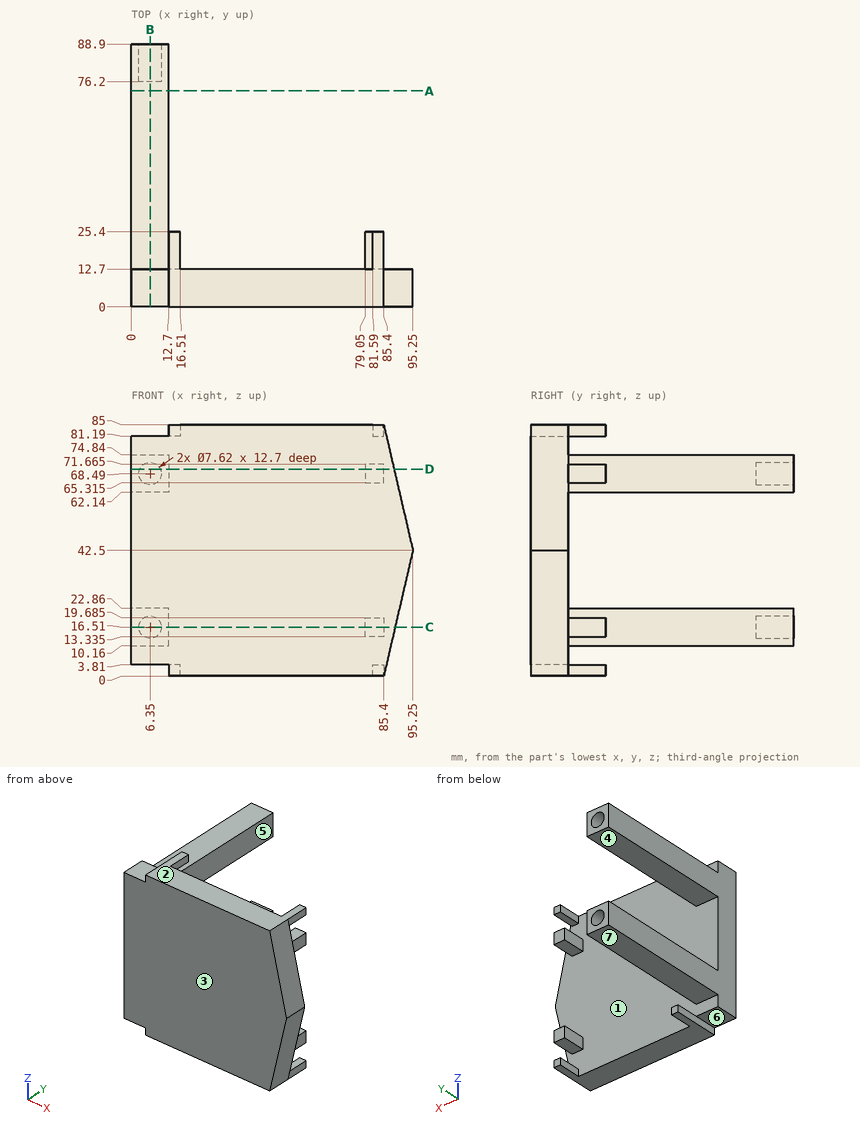
Answer from the drawing. Dimensions are ordinates in mm from the lowest x, y and z of the part. A direction names the side the tool comes from. Give positions to 0.01 mm unless a question says otherwise; leave off trailing zeros. Write each loop counter-clockwise with the first axis right and the second up, starting at its lowest first coordinate (ties: lowest second). Pieces come first, ordered by that corner, then holes.
1) A tool of negligible diameter and unlimited length cuts with its end or side. For the marked faces 5, 6 and 7, from which of +Z, -Z, +X, -X, +Y, -Y can it reach the whole face along a straight path? Write none if from no direction.
2) Section B-B (x = 6.35) is taken. Write down the section's boundary in (y, z), and give its area (3 significant figures).
3) Section D-D (z = 70) is taken. Write down the section's boundary in (x, y).
4) Section A-A (y = 73) is taken. Write down the section's boundary in (x, z).
5) For a pull along Z with two mould halves and no side action, classify the marked faces 1, 2, 3 and 4 as pulls with the +Z half, pulls with the -Z half, needs draft (parallel to the pull), parting line crosses it, or undercut.
6) Find the intervals of material crossed by L1, parallel to Z at x = 6, y = 83; L2, parallel to X at y = 83, z = 68; L3, parallel to Y at x = 37, z = 55.5, in increasing order.
7) Section C-C (z = 16.51) is taken. Write down the section's boundary in (x, y), and give its area (3 significant figures).
8) Given P1, Ø6, axis at x = 7.5, z = 16, coming from the +Y side; P2, Ø10, axis at x = 8, y = 39.5, coming from the -Z side; P3, Ø3, axis at x = 57, z = 21, coming from the +Y side; P4, Ø1.9, axis at y = 21.5, z = 83, coming from the -X side, each flat-ended and moving along its own axis, determine where each tip first touches the part or whether it passes through.
Response:
1. face 5: +Y
1. face 6: -Z, -X, +Y, -Y
1. face 7: -Z, +X, -X, +Y
2. outline: (0, 3.81) - (12.7, 3.81) - (12.7, 10.16) - (88.9, 10.16) - (88.9, 12.7) - (76.2, 12.7) - (76.2, 20.32) - (88.9, 20.32) - (88.9, 22.86) - (12.7, 22.86) - (12.7, 62.14) - (88.9, 62.14) - (88.9, 64.68) - (76.2, 64.68) - (76.2, 72.3) - (88.9, 72.3) - (88.9, 74.84) - (12.7, 74.84) - (12.7, 81.19) - (0, 81.19) - close
2. area: 2,720 mm2
3. outline: (0, 0) - (88.88, 0) - (88.88, 12.7) - (85.4, 12.7) - (85.4, 25.4) - (79.05, 25.4) - (79.05, 12.7) - (12.7, 12.7) - (12.7, 88.9) - (9.85, 88.9) - (9.85, 76.2) - (2.85, 76.2) - (2.85, 88.9) - (0, 88.9) - close
4. outline: (0, 10.16) - (12.7, 10.16) - (12.7, 22.86) - (0, 22.86) - close; (0, 62.14) - (12.7, 62.14) - (12.7, 74.84) - (0, 74.84) - close
5. face 1: undercut
5. face 2: pulls with the +Z half
5. face 3: needs draft
5. face 4: undercut
6. L1: z = 10.16 to 12.72, 20.3 to 22.86, 62.14 to 64.7, 72.28 to 74.84
6. L2: x = 0 to 2.57, 10.13 to 12.7
6. L3: y = 0 to 12.7
7. outline: (0, 0) - (89.23, 0) - (89.23, 12.7) - (85.4, 12.7) - (85.4, 25.4) - (79.05, 25.4) - (79.05, 12.7) - (12.7, 12.7) - (12.7, 88.9) - (10.16, 88.9) - (10.16, 76.2) - (2.54, 76.2) - (2.54, 88.9) - (0, 88.9) - close
7. area: 2,080 mm2
8. P1: stops at y = 88.9
8. P2: stops at z = 10.16
8. P3: stops at y = 12.7
8. P4: stops at x = 12.7
